Verification items for the finished model (mm, model axes). Give positions to 0.01 mm unless a question says otherwise; leave off trailing zeros. Order: outer loops, then holes, each group sorted by start corner. A loop starts at its lowest first (then second) coordinate and runs counter-clockwise, first axis right, second up.
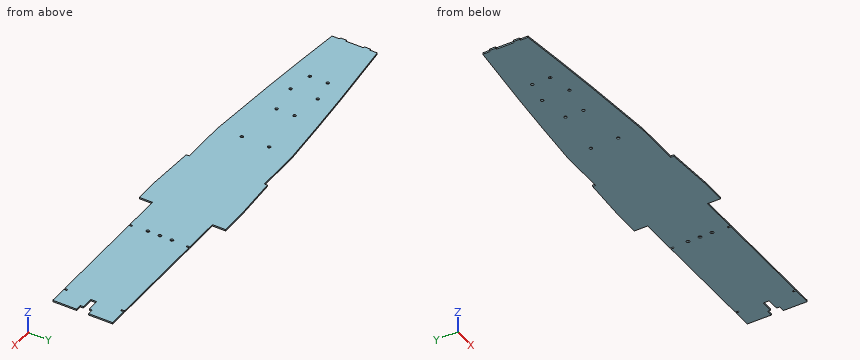
from build123d import *

# Parameters (mm, degrees)
BOSS_EXTRUDE1_DEPTH    = 1.5875
SKETCH10_W             = 6.35
SKETCH10_H             = 68.58
CUT_EXTRUDE5_DEPTH     = 637.645771754
CUT_EXTRUDE1_DEPTH     = 631.312352085
SKETCH4_W              = 1.5875
SKETCH4_H              = 3.175
CUT_EXTRUDE2_DEPTH     = 631.312352085
SKETCH6_W              = 47.338109293
SKETCH6_H              = 3.175
CUT_EXTRUDE3_DEPTH     = 631.312352085
SKETCH7_R              = 1.5875
ARTS4_MOUNT_DEPTH      = 631.312352085
SKETCH8_R              = 1.5875
TELEMETRUM_MOUNT_DEPTH = 631.312352085
SKETCH9_R              = 1.74625
CUT_EXTRUDE4_DEPTH     = 631.312352085


with BuildPart() as part:
    # Sketch1 → Boss-Extrude1 (new body)
    with BuildSketch(Plane.XY):
        with BuildLine():
            Line((508, -45.72), (508, -34.29))
            Line((508, -34.29), (635, -34.29))
            Line((635, -34.29), (635, 34.29))
            Line((635, 34.29), (508, 34.29))
            Line((508, 34.29), (508, 45.72))
            Line((508, 45.72), (429.947642932, 45.72))
            add(Edge.make_bspline(
                [(161.29, 23.981640211), (161.616784041, 24.018741883), (172.383373415, 25.239568053), (204.048179593, 28.679227521), (256.348102033, 33.727983978), (319.188209115, 38.915614913), (371.60802888, 42.52482202), (408.536828327, 44.644949518), (424.488578703, 45.455997775), (429.947642932, 45.72)],
                knots=[0.31962734, 0.31962734, 0.31962734, 0.31962734, 0.321557959, 0.383234508, 0.506587607, 0.629940705, 0.753293803, 0.814970352, 0.847054623, 0.847054623, 0.847054623, 0.847054623], degree=3))
            Line((161.29, 23.981640211), (161.29, 15.875))
            Line((161.29, 15.875), (159.7025, 15.875))
            Line((159.7025, 15.875), (159.7025, 9.525))
            Line((159.7025, 9.525), (161.29, 9.525))
            Line((161.29, 9.525), (161.29, -9.525))
            Line((161.29, -9.525), (159.7025, -9.525))
            Line((159.7025, -9.525), (159.7025, -15.875))
            Line((159.7025, -15.875), (161.29, -15.875))
            Line((161.29, -15.875), (161.29, -23.981640211))
            add(Edge.make_bspline(
                [(429.947642932, -45.72), (424.488578703, -45.455997775), (408.536828327, -44.644949518), (371.60802888, -42.52482202), (319.188209115, -38.915614913), (256.348102033, -33.727983978), (204.048179593, -28.679227521), (172.383373415, -25.239568053), (161.616784041, -24.018741883), (161.29, -23.981640211)],
                knots=[0.16612059, 0.16612059, 0.16612059, 0.16612059, 0.198204861, 0.25988141, 0.383234508, 0.506587607, 0.629940705, 0.691617254, 0.693547873, 0.693547873, 0.693547873, 0.693547873], degree=3))
            Line((429.947642932, -45.72), (508, -45.72))
        make_face()
    extrude(amount=BOSS_EXTRUDE1_DEPTH)

    # Sketch10 → Cut-Extrude5 (cut, through all)
    with BuildSketch(Plane(origin=(0, 0, 0), x_dir=(-1, 0, 0), z_dir=(0, 0, -1))):
        with Locations((-631.825, 0)):
            Rectangle(SKETCH10_W, SKETCH10_H)
    extrude(amount=-CUT_EXTRUDE5_DEPTH, mode=Mode.SUBTRACT)

    # Sketch3 → Cut-Extrude1 (cut, through all)
    with BuildSketch(Plane.XY.offset(1.5875)):
        Polygon((635, 34.29), (508, 34.29), (508, 45.72), (457.2, 45.72), (457.2, 31.75), (635, 31.75), align=None)
        Polygon((508, -45.72), (508, -34.29), (635, -34.29), (635, -31.75), (457.2, -31.75), (457.2, -45.72), align=None)
        Polygon((622.3, 6.35), (622.3, 3.175), (609.6, 3.175), (609.6, -3.175), (622.3, -3.175), (622.3, -6.35), (628.65, -6.35), (628.65, 6.35), align=None)
    extrude(amount=-CUT_EXTRUDE1_DEPTH, mode=Mode.SUBTRACT)

    # Sketch4 → Cut-Extrude2 (cut, through all)
    with BuildSketch(Plane.XY.offset(1.5875)):
        with Locations((496.7605, 30.1625)):
            Rectangle(SKETCH4_W, SKETCH4_H)
        with Locations((608.80625, 30.1625)):
            Rectangle(SKETCH4_W, SKETCH4_H)
        with Locations((496.7605, -30.1625)):
            Rectangle(SKETCH4_W, SKETCH4_H)
        with Locations((608.80625, -30.1625)):
            Rectangle(SKETCH4_W, SKETCH4_H)
    extrude(amount=-CUT_EXTRUDE2_DEPTH, mode=Mode.SUBTRACT)

    # Sketch6 → Cut-Extrude3 (cut, through all)
    with BuildSketch(Plane.XY.offset(1.5875)):
        with Locations((357.330945353, 41.432202354)):
            Rectangle(SKETCH6_W, SKETCH6_H)
        with Locations((357.330945353, -41.432202354)):
            Rectangle(SKETCH6_W, SKETCH6_H)
    extrude(amount=-CUT_EXTRUDE3_DEPTH, mode=Mode.SUBTRACT)

    # Sketch7 → ARTS4 mount (cut, through all)
    with BuildSketch(Plane.XY.offset(1.5875)):
        with Locations((331.688780886, 14.478)):
            Circle(SKETCH7_R)
        with Locations((331.688780886, -14.478)):
            Circle(SKETCH7_R)
        with Locations((247.868780886, 14.478)):
            Circle(SKETCH7_R)
        with Locations((247.868780886, -14.478)):
            Circle(SKETCH7_R)
    extrude(amount=-ARTS4_MOUNT_DEPTH, mode=Mode.SUBTRACT)

    # Sketch8 → Telemetrum Mount (cut, through all)
    with BuildSketch(Plane.XY.offset(1.5875)):
        with Locations((280.018433255, 9.525)):
            Circle(SKETCH8_R)
        with Locations((280.018433255, -9.525)):
            Circle(SKETCH8_R)
        with Locations((222.893833255, -9.525)):
            Circle(SKETCH8_R)
        with Locations((222.893833255, 9.525)):
            Circle(SKETCH8_R)
    extrude(amount=-TELEMETRUM_MOUNT_DEPTH, mode=Mode.SUBTRACT)

    # Sketch9 → Cut-Extrude4 (cut, through all)
    with BuildSketch(Plane.XY.offset(1.5875)):
        with Locations((495.96675, -12.7)):
            Circle(SKETCH9_R)
        with Locations((495.96675, 12.7)):
            Circle(SKETCH9_R)
        with Locations((495.96675, 0)):
            Circle(SKETCH9_R)
    extrude(amount=-CUT_EXTRUDE4_DEPTH, mode=Mode.SUBTRACT)


solid = part.part
(1) Scan lines: line 1 (Y direction, x = 486, z = 0.2); line 2 (X direction, y = -4, z = 0.9); line 3 (Y direction, x = 360, z = 1.2). Record each from-to range of solid material in increasing order.
Solved:
line 1: y = -31.75 to 31.75
line 2: x = 161.29 to 622.3
line 3: y = -39.84 to 39.84
(2) Section check A-A, the plane x = 509.5. Enter the section's corners in (y, z).
Solved:
outline: (-31.75, 0) - (31.75, 0) - (31.75, 1.59) - (-31.75, 1.59) - close
(3) Go/stop test with flat-tipped pins: pin 1 (0.8 mm diameter, centred on x = 160.5, z = 0.5, fed in from +Y) (3 decimals); pin 2 (0.5 mm diameter, centred on y = -4, z = 0.5, fed in from +X); pin 3 (0.8 mm diameter, centred on x = 472.5, z = 1, fed in from -Y). Record where each tip stops, or that it passes through.
Solved:
pin 1: stops at y = 15.875
pin 2: stops at x = 622.3
pin 3: stops at y = -31.75
(4) Section check B-B, the plane z = 0.95. Give the number of separate pieces and of enclosed holes in the cut face, then the cut area to 3 significant figures.
Solved:
separate pieces: 1
enclosed holes: 11
area: 32,400 mm2
